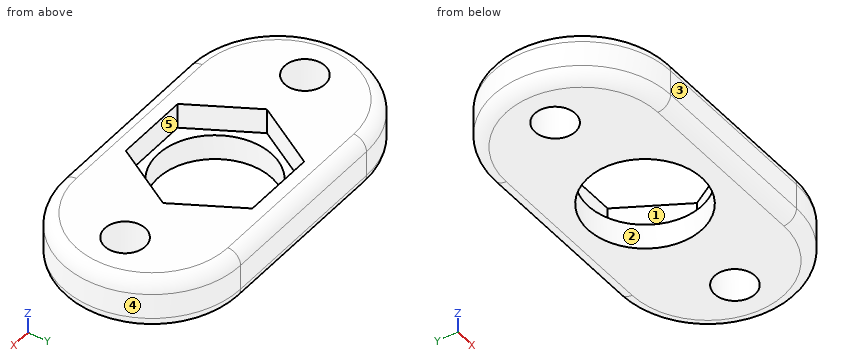
```python
from build123d import *

# Parameters (mm, degrees)
BOSS_EXTRU_1_DEPTH      = 4
ESQUISSE3_R             = 4.5
ESQUISSE3_R_2           = 1.6
ENL_V_MAT_EXTRU_1_DEPTH = 5
ENL_V_MAT_EXTRU_2_DEPTH = 2
CONG_1_R                = 1


with BuildPart() as part:
    # Esquisse1 → Boss.-Extru.1 (new body)
    with BuildSketch(Plane.XY):
        with BuildLine():
            Line((-27.254178511, 7), (-13.254178511, 7))
            ThreePointArc((-13.254178511, 7), (-6.254178511, 0), (-13.254178511, -7))
            Line((-13.254178511, -7), (-27.254178511, -7))
            ThreePointArc((-27.254178511, -7), (-34.254178511, 0), (-27.254178511, 7))
        make_face()
    extrude(amount=BOSS_EXTRU_1_DEPTH)

    # Esquisse3 → Enlèv. mat.-Extru.1 (cut, through all)
    with BuildSketch(Plane.XY.offset(4)):
        with Locations((-20.254178511, 0)):
            Circle(ESQUISSE3_R)
        with Locations((-30.254178511, 0)):
            Circle(ESQUISSE3_R_2)
        with Locations((-10.254178511, 0)):
            Circle(ESQUISSE3_R_2)
    extrude(amount=-ENL_V_MAT_EXTRU_1_DEPTH, mode=Mode.SUBTRACT)

    # Esquisse4 → Enlèv. mat.-Extru.2 (cut)
    with BuildSketch(Plane.XY.offset(4)):
        Polygon((-23.140929857, 5), (-26.027681203, 0), (-23.140929857, -5), (-17.367427165, -5), (-14.480675819, 0), (-17.367427165, 5), align=None)
    extrude(amount=-ENL_V_MAT_EXTRU_2_DEPTH, mode=Mode.SUBTRACT)

    # Congé1
    cong_1_edges = [part.edges().sort_by_distance(p)[0] for p in [
        (-6.254178511, 0, 4),
        (-20.254178511, 7, 4),
        (-34.254178511, 0, 4),
        (-20.254178511, 7, 0),
        (-6.254178511, 0, 0),
        (-20.254178511, -7, 0),
        (-34.254178511, 0, 0),
        (-20.254178511, -7, 4),
    ]]
    fillet(cong_1_edges, radius=CONG_1_R)


solid = part.part
```
Check sheet for the modelled part. Datum: model origin and axes. Units: mm. Face numbers are marked on the shaded views. A direction names the side the tool comes from. Coordinates: 2 decimals unless noted, no trailing zeros. Order: outer loops, then holes, each group sorted by start corner. A loop starts at its lowest first (then second) coordinate and runs counter-clockwise, first axis right, second up. Notation, with made-up numbers: M 4,-38.5 L 63,-38.5 A12 ccw 63,-21.5 Z; hole C 38.5,83 d5. An arc over 180 degrees is marked long. One line per question, with ' | ' between items. Start each with the question number.
Item 1: Sectioned sample at C-C on x = -25.25. Record the cut outline in (y, z), and give its area (3 significant figures).
Item 2: Material ranges on line 1 (Y direction, x = -20.5, z = 3.1); line 2 (X direction, y = -0.75, z = 2.9); line 3 (Y direction, x = -17.75, z = 3.6), recorded low to high.
Item 3: Sectioned sample at B-B on z = 0.45. Record the cut outline in (x, y).
Item 4: Mould release check, pull along Y, two halves, no side actions. Record for the marked faces 3, 4 and 5: pulls with the +Y half, pulls with the -Y half, needs draft (parallel to the pull), parting line crosses it, or undercut.
Item 5: Sectioned sample at A-A on x = -17.75. Record the cut outline in (y, z), and give its area (3 significant figures).
Item 6: Gauge pin test, flat end, axial feed: P1, Ø1.5, axis at x = -29, z = 3, coming from the -Y side. Record the tip position at first contact, or that the pin passes through.
Item 7: Access from +Z, -Z, +X, -X, +Y, -Y to the whole of each face (thin tool, end or side, straight path). Record for the marked faces 1 and 2.
Answer below:
1) outline: M -7,1 A1 ccw -6,0 L 6,0 A1 ccw 7,1 L 7,3 A1 ccw 6,4 L 1.35,4 L 1.35,2 L -1.35,2 L -1.35,4 L -6,4 A1 ccw -7,3 Z | area: 49.8 mm^2
2) line 1: y = -6.99 to -5, 5 to 6.99 | line 2: x = -34.21 to -31.67, -28.84 to -25.59, -14.91 to -11.67, -8.84 to -6.29 | line 3: y = -6.8 to -5, 5 to 6.8
3) outline: M -27.25,-6.84 L -13.25,-6.84 A6.84 ccw -13.25,6.84 L -27.25,6.84 A6.84 ccw Z; hole C -30.25,0 d3.2; hole C -20.25,0 d9; hole C -10.25,0 d3.2
4) face 3: pulls with the -Y half | face 4: parting line crosses it | face 5: undercut
5) outline: M -7,1 A1 ccw -6,0 L -3.74,0 L -3.74,2 L -5,2 L -5,4 L -6,4 A1 ccw -7,3 Z; M 3.74,0 L 6,0 A1 ccw 7,1 L 7,3 A1 ccw 6,4 L 5,4 L 5,2 L 3.74,2 Z | area: 20.2 mm^2
6) P1: stops at y = -6.93
7) face 1: +Z | face 2: +Z, -Z
